Check sheet for the modelled part. Datum: model origin and axes. Units: mm. A direction names the side the tool comes from. Round coordinates to 2 decimals unless told otherwise and drop trailing zeros. Order: outer loops, then holes, each group sorted by start corner. A loop starts at its lowest first (then second) coordinate and runs counter-clockwise, first axis right, second up.
(1) Tool access check on faces 4 (the flat face through (-21.45, 1, -5)), 5 (the flat face through (22, 8, 5.855)), 6 (the flat face through (-17.45, 3, 0)), 7 (the flat face through (22, 10.5, 0)). Record the directions out of +Z, -Z, +X, -X, +Y, -Y that give a thin tool (end or side, any length) a straight path to the whole face; none if there is none.
(2) Sectioned sample at D-D, the plane z = 6.75. Enter the section's corners in (x, y), and give its area (3 significant figures).
(3) Sectioned sample at A-A, the plane z = 0. Enter the section's corners in (x, y).
(4) Mould release check, pull along Z, two halves, no side actions. Record for faces 1 (the flat face through (22, 6.5, 0)), 2 (the cylindrical face through (21.165, 2.301, -0.126)), 3 (the flat face through (22, 8, -5.887)): released by +Z, released by -Z, zero draft, split by the parting line, or undercut.
(5) Sectioned sample at C-C, the plane y = 11.25. Enter the section's corners in (x, z).
(6) Sectioned sample at B-B, the plane x = -2.45. Enter the section's corners in (y, z).
(7) Thickness scan on probe 1 along Z at (x, y) = (-2.45, 0.4); probe 2 along X at (y, z) = (0.2, 0); probe 3 along Z at (x, y) = (21.5, 6.75). Record the ranges inside material, lowest first.
(8) Depth check by flat-ended pin: pin 1 (1 mm diameter, centred on y = 0.5, z = 4.5, fed in from -X); pin 2 (5.5 mm diameter, centred on x = -9, z = -0.5, fed in from +Y); pin 3 (1.2 mm diameter, centred on x = -20.5, z = 0, fed in from +Y); pin 4 (0.8 mm diameter, centred on x = 22.5, z = 0.5, fed in from -Y). Enter the tip coordinate at first touch or a pass-through.
Autodesk Inventor part; units mm, degrees
ref_plane "YZ Plane" through (0, 0, 0) normal (1, 0, 0) x (0, 1, 0)
ref_plane "XZ Plane" through (0, 0, 0) normal (0, 1, 0) x (-1, 0, 0)
ref_plane "XY Plane" through (0, 0, 0) normal (0, 0, 1) x (1, 0, 0)
sketch "Esquisse1" plane through (0, 0, 0) normal (0, 1, 0) x (-1, 0, 0)
  line L0 (21.45, 8.8) -> (-21.45, 8.8)
  line L1 (-21.45, 8.8) -> (-21.45, -8.8)
  line L2 (-21.45, -8.8) -> (21.45, -8.8)
  line L3 (21.45, -8.8) -> (21.45, 8.8)
  line L4 (21.45, 8.8) -> (-21.45, -8.8) construction
  line L5 (-21.45, 8.8) -> (21.45, -8.8) construction
  point P0 (0, 0)
  dimension "d0" = 42.9
  dimension "d1" = 17.6
extrude "Extrusion1" add sketch "Esquisse1" along normal blind 2
sketch "Esquisse2" plane through (21.45, 0, 8.8) normal (1, 0, 0) x (0, 0, -1)
  line L0 (4.6867, 10.5) -> (12.6867, 10.5)
  line L1 (12.6867, 10.5) -> (12.6867, 6.5)
  line L2 (12.6867, 6.5) -> (4.6867, 6.5)
  line L3 (4.6867, 6.5) -> (4.6867, 10.5)
  line L4 (4.6867, 10.5) -> (12.6867, 6.5) construction
  line L5 (12.6867, 10.5) -> (4.6867, 6.5) construction
  line L6 (2.9446, 12.5) -> (14.6867, 12.5)
  line L7 (14.6867, 12.5) -> (14.6867, 4.3203)
  line L8 (2.9446, 4.6719) -> (2.9446, 12.5)
  line L9 (2.9446, 12.5) -> (14.6867, 4.3203) construction
  line L10 (14.6867, 12.5) -> (2.9446, 4.6719) construction
  line L11 (0, 2) -> (17.6, 2)
  line L12 (2.9446, 4.6719) -> (2.9446, 0)
  line L13 (0, 0) -> (17.6, 0)
  line L14 (14.6867, 4.3203) -> (14.6867, 0)
  line L15 (2.9446, 0) -> (14.6867, 0)
  point P0 (8.8, 0)
  point P1 (8.6867, 8.5)
  point P2 (8.6867, 8.5)
  dimension "d4" = 4.5
  dimension "d6" = 2
  dimension "d7" = 8
  dimension "d8" = 4
extrude "Extrusion2" add sketch "Esquisse2" along normal blind 1.5
sketch "Esquisse4" plane through (0, 2, 0) normal (0, 1, 0) x (1, 0, 0)
  line L0 (-21.45, 8.8) -> (-21.45, -8.8)
  point P0 (0, 0)
  point P1 (-2.45, 0)
  dimension "d18" = 19
hole "Perçage2" at (-2.45, 2, 0) direction (0, -1, 0) diameter 4 end through all countersink diameter 6 countersink angle 90
sketch "Esquisse5" plane through (21.45, 0, 8.8) normal (1, 0, 0) x (0, 0, -1)
  line L0 (0, 0) -> (2.9446, 0)
  line L1 (2.9446, 2) -> (14.6867, 2)
  line L2 (0, 0) -> (2.9446, 0)
  line L3 (2.9446, 0) -> (2.9446, 2)
  line L4 (2.9446, 2) -> (0, 2)
  line L5 (0, 2) -> (0, 0)
  line L6 (2.9446, 0) -> (14.6867, 0)
  line L7 (14.6867, 2) -> (17.6, 2)
  line L8 (14.6867, 0) -> (17.6, 0)
  line L9 (17.6, 0) -> (17.6, 2)
  line L10 (17.6, 2) -> (14.6867, 2)
  line L11 (14.6867, 2) -> (14.6867, 0)
  point P0 (8.8, 0)
extrude "Extrusion3" add sketch "Esquisse5" along normal up to surface (1.5 mm away) contours L5 L4 L3 L0 | L11 L7 L9 L8
fillet "Congé1" radius 2 2 edges at (22.2, 2, 5.8554) (22.2, 2, -5.8867)
fillet "Congé2" radius 1 1 edges at (21.45, 2, -0.0157)
sketch "Esquisse6" plane through (0, 0, 0) normal (0, -1, 0) x (1, 0, 0)
  circle A0 centre (-23.45, 0) radius 2
  line L0 (-21.45, -8.8) -> (-21.45, 8.8)
  line L1 (-23.45, 2) -> (-17.45, 2)
  line L2 (-17.45, 2) -> (-17.45, -2)
  line L3 (-17.45, -2) -> (-23.45, -2)
  line L4 (0, 0) -> (4.0498, 0)
  dimension "d30" = 4
  dimension "d31" = 4
extrude "Extrusion4" add sketch "Esquisse6" against normal blind 4.8
sketch "Esquisse7" plane through (0, 4.8, 0) normal (0, 1, 0) x (1, 0, 0)
  circle A0 centre (-23.45, 0) radius 2
  arc A1 (-23.45, 2) -> (-23.45, -2) centre (-23.45, 0) ccw
  point P0 (0, 0)
extrude "Extrusion5" add sketch "Esquisse7" along normal blind 1.7
equation "\"d6\" = d5"
properties part number "arduino_holder"
Derived:
1. face 4: -Z, -X, +Y, -Y
1. face 5: +Z, +X, -X, +Y
1. face 6: +Z, -Z, +Y
1. face 7: +X, -X
2. outline: (-21.45, 0) - (22.95, 0) - (22.95, 2.33) - (21.2, 2.33) arc R1 cw to (20.45, 2) - (-21.45, 2) - close
2. area: 89.5 mm2
3. outline: (-25.45, 0) - (-4.45, 0) - (-4.45, 1) - (-5.45, 2) - (-17.45, 2) - (-17.45, 4.8) - (-21.45, 4.8) - (-21.45, 6.5) - (-25.45, 6.5) - close; (-0.45, 0) - (22.95, 0) - (22.95, 6.5) - (21.45, 6.5) - (21.45, 3) arc R1 cw to (20.45, 2) - (0.55, 2) - (-0.45, 1) - close; (21.45, 10.5) - (22.95, 10.5) - (22.95, 12.5) - (21.45, 12.5) - close
4. face 1: undercut
4. face 2: zero draft
4. face 3: released by -Z
5. outline: (21.45, -5.89) - (22.95, -5.89) - (22.95, 5.86) - (21.45, 5.86) - close
6. outline: (0, -8.8) - (2, -8.8) - (2, -3) - (1, -2) - (0, -2) - close; (0, 2) - (1, 2) - (2, 3) - (2, 8.8) - (0, 8.8) - close
7. probe 1: z = -8.8 to -2, 2 to 8.8
7. probe 2: x = -25.45 to -4.45, -0.45 to 22.95
7. probe 3: z = -5.89 to -3.89, 4.11 to 5.86
8. pin 1: stops at x = -21.45
8. pin 2: stops at y = 2
8. pin 3: stops at y = 4.8
8. pin 4: stops at y = 0
